For this review, take the finished solid that the model builds, in its own axes (mm). A direction names the side the tool comes from. Round coordinates to 2 decimals unless told otherwise and drop trailing zeros. Write each loop counter-clockwise with the first axis right and the second up, starting at its lowest first coordinate (ties: lowest second). Pieces come first, ordered by that corner, then holes. Notation, with made-up numbers: M 33,75 L 90,75 A31 ccw 90,104 Z; hole C 24.5,89.5 d11. An arc over 180 degrees is marked long. Answer in a Markdown table with one row per item.
```python
from build123d import *

# Parameters (mm, degrees)
SKETCH1_R           = 1.5
BOSS_EXTRUDE1_DEPTH = 4
CUT_EXTRUDE1_START  = -4
CUT_EXTRUDE1_DEPTH  = 4
CIRPATTERN2_COUNT   = 11
SKETCH3_W           = 6.093608585
SKETCH3_H           = 4.996234569
BOSS_EXTRUDE2_DEPTH = 4
SKETCH4_R           = 2.5
CUT_EXTRUDE2_DEPTH  = 4


with BuildPart() as part:
    # Sketch1 → Boss-Extrude1 (new body)
    with BuildSketch(Plane.XY):
        with BuildLine():
            Line((-18, 2.5), (12.545643943, 2.5))
            ThreePointArc((12.545643943, 2.5), (24, 0), (12.545643943, -2.5))
            Line((12.545643943, -2.5), (-18, -2.5))
            ThreePointArc((-18, -2.5), (-20.5, 0), (-18, 2.5))
        make_face()
        with Locations((-18, 0)):
            Circle(SKETCH1_R, mode=Mode.SUBTRACT)
    extrude(amount=BOSS_EXTRUDE1_DEPTH)

    # Sketch2 → Cut-Extrude1 (cut)
    with BuildSketch(Plane.XY.offset(4).offset(CUT_EXTRUDE1_START)):
        with BuildLine():
            Line((18.72, 5.06), (18.653012702, 4.81))
            ThreePointArc((18.653012702, 4.81), (19.291515108, 4.181419291), (19.930017513, 4.81))
            ThreePointArc((19.930017513, 4.81), (19.930088137, 4.81213776), (19.930232945, 4.814271778))
            ThreePointArc((19.930232945, 4.814271778), (20.377650935, 5.25023041), (21, 5.196152423))
            ThreePointArc((21, 5.196152423), (19.552914271, 5.795554958), (18, 6))
            ThreePointArc((18, 6), (18.589879661, 5.706078038), (18.72, 5.06))
        make_face()
    cut_extrude1 = extrude(amount=CUT_EXTRUDE1_DEPTH, mode=Mode.SUBTRACT)

    # CirPattern2: Cut-Extrude1 ×11 about axis
    cirpattern2_axis = Axis((18, 0, 0), (0, 0, 1))
    for i in range(1, CIRPATTERN2_COUNT):
        add(cut_extrude1.rotate(cirpattern2_axis, i * 360 / CIRPATTERN2_COUNT), mode=Mode.SUBTRACT)

    # Sketch3 → Boss-Extrude2 (add)
    with BuildSketch(Plane.XY.offset(4)):
        with Locations((12.072309907, 0.001882715)):
            Rectangle(SKETCH3_W, SKETCH3_H)
    extrude(amount=-BOSS_EXTRUDE2_DEPTH)

    # Sketch4 → Cut-Extrude2 (cut)
    with BuildSketch(Plane.XY.offset(4)):
        with Locations((17.976309792, 0.185764476)):
            Circle(SKETCH4_R)
    extrude(amount=-CUT_EXTRUDE2_DEPTH, mode=Mode.SUBTRACT)


solid = part.part
```
Q1. Take a section at A-A (y = 0.75). State the section outline as (x, z) points.
Found:
| item | result |
|---|---|
| outline | M -20.38,0 L -19.3,0 L -19.3,4 L -20.38,4 Z; M -16.7,0 L 15.54,0 L 15.54,4 L -16.7,4 Z; M 20.41,0 L 22.29,0 L 22.29,4 L 20.41,4 Z |
Q2. Take a section at C-C (z = 0.65). State how many separate pieces and enclosed holes the cut face has, then the cut area to 3 significant figures.
Found:
| item | result |
|---|---|
| separate pieces | 1 |
| enclosed holes | 2 |
| area | 226 mm² |
Q3. Take a section at B-B (x = 11). State the section outline as (y, z) points, then the cut area to 3 significant figures.
Found:
| item | result |
|---|---|
| outline | M -2.5,0 L 2.5,0 L 2.5,4 L -2.5,4 Z |
| area | 20.0 mm² |
Q4. Insertion check: P1, Ø1, axis at y = 2, z = 1, coming from the -X side; P2, Ø4, axis at x = 17.98, y = 0.19, coming from the +Z side; P3, Ø1, axis at y = 0.5, z = 1.5, coming from the +X side; P4, Ø1.7, axis at x = 13.5, z = 3, coming from the -Y side. Each pin has a flat end and moves straight along its axis. Give the tip position at first contact, or say it passes through.
Found:
| item | result |
|---|---|
| P1 | x = -20 |
| P2 | through |
| P3 | x = 23.78 |
| P4 | y = -4.37 |
Q5. Mouldability with a two-part tool opening along X and no side actions: class faces 1 (the face through (21.58, 4.49, 1.97)), 2 (the face through (20.369, 5.247, 1.972)), 3 (the face through (13.3, -3.3, 2)) as +X half, -X half, draft (parallel to the pull), parting line (faces both ways), or undercut.
Found:
| item | result |
|---|---|
| face 1 | +X half |
| face 2 | undercut |
| face 3 | -X half |
Q6. Machinability: for faces 4 (the face through (-3, 2.5, 2)), 5 (the face through (20.414, -5.227, 1.972)), 6 (the face through (19.28, 4.18, 1.97)), which of the approach directions +Z, -Z, +X, -X, +Y, -Y give a long, thin tool a straight path to every point of the face, cutting with its end or side? Answer none if there is none.
Found:
| item | result |
|---|---|
| face 4 | +Z, -Z, -X, +Y |
| face 5 | +Z, -Z, +X |
| face 6 | +Z, -Z |
Q7. For probe 1 along X at (y, z) = (0.75, 1.45); probe 2 along X at (y, z) = (-0.5, 3.55); probe 3 along Y at (x, z) = (-18, 1.7), list the stretches that pass through material, from the lowest coordinate up.
Found:
| item | result |
|---|---|
| probe 1 | -20.38 to -19.3, -16.7 to 15.54, 20.41 to 22.29 |
| probe 2 | -20.45 to -19.41, -16.59 to 15.57, 20.38 to 23.98 |
| probe 3 | -2.5 to -1.5, 1.5 to 2.5 |
